from build123d import *

# Parameters (mm, degrees)
BOSS_EXTRUDE1_DEPTH = 22.86
SKETCH2_R           = 3.175
CUT_EXTRUDE1_DEPTH  = 50.737325059
SKETCH3_R           = 4.365625
CUT_EXTRUDE2_DEPTH  = 23.622


with BuildPart() as part:
    # Sketch1 → Boss-Extrude1 (new body)
    with BuildSketch(Plane(origin=(0, 0, 0), x_dir=(1, 0, 0), z_dir=(0, 1, 0))):
        Polygon((-11.176, -25.4), (-8.89, -25.4), (-8.89, 25.4), (8.89, 25.4), (8.89, -25.4), (11.176, -25.4), (11.176, 38.1), (-11.176, 38.1), align=None)
    extrude(amount=BOSS_EXTRUDE1_DEPTH)

    # Sketch2 → Cut-Extrude1 (cut, through all)
    with BuildSketch(Plane(origin=(11.176, 0, 0), x_dir=(0, 0, -1), z_dir=(1, 0, 0))):
        with Locations((-12.7, 11.43)):
            Circle(SKETCH2_R)
    extrude(amount=-CUT_EXTRUDE1_DEPTH, mode=Mode.SUBTRACT)

    # Sketch3 → Cut-Extrude2 (cut)
    with BuildSketch(Plane(origin=(0, 0, -38.1), x_dir=(-1, 0, 0), z_dir=(0, 0, -1))):
        with Locations((0, 11.43)):
            Circle(SKETCH3_R)
    extrude(amount=-CUT_EXTRUDE2_DEPTH, mode=Mode.SUBTRACT)


solid = part.part
CAD build for the part. Positions are in the model's coordinates, mm. A direction names the side the tool comes from. Give positions to 0.01 mm unless a question says otherwise; leave off trailing zeros. Order: outer loops, then holes, each group sorted by start corner. A loop starts at its lowest first (then second) coordinate and runs counter-clockwise, first axis right, second up. Notation, with made-up numbers: (15.5, 43) -> (40.5, 43) arc R31 ccw to (40.5, 74) -> close; hole circle Ø1 at (-17.75, 78.25). An arc over 180 degrees is marked (long way). Return JSON: item names as keys, results as strings.
Q1. Saw through at A-A (z = 12.7). Write the cut outline in (x, y) (3 decimals), then the cut area to 3 significant figures.
Working result:
{"outline": "(-11.176, 0) -> (-8.89, 0) -> (-8.89, 8.255) -> (-11.176, 8.255) -> close; (-11.176, 14.605) -> (-8.89, 14.605) -> (-8.89, 22.86) -> (-11.176, 22.86) -> close; (8.89, 0) -> (11.176, 0) -> (11.176, 8.255) -> (8.89, 8.255) -> close; (8.89, 14.605) -> (11.176, 14.605) -> (11.176, 22.86) -> (8.89, 22.86) -> close", "area": "75.5 mm²"}
Q2. Saw through at C-C (x = 0). Write the cut outline in (y, z).
Working result:
{"outline": "(0, -38.1) -> (7.06, -38.1) -> (7.06, -25.4) -> (0, -25.4) -> close; (15.8, -38.1) -> (22.86, -38.1) -> (22.86, -25.4) -> (15.8, -25.4) -> close"}
Q3. Saw through at D-D (z = 4.5). Write the cut outline in (x, y), then the cut area to 3 significant figures.
Working result:
{"outline": "(-11.18, 0) -> (-8.89, 0) -> (-8.89, 22.86) -> (-11.18, 22.86) -> close; (8.89, 0) -> (11.18, 0) -> (11.18, 22.86) -> (8.89, 22.86) -> close", "area": "105 mm²"}
Q4. Mould opens along Y. For faces 1 (the face through (0, 22.86, -28)), 2 (the face through (-10.02, 12.38, 9.67)), 3 (the face through (8.89, 11, 0)) say: pulls with the +Y half, pulls with the -Y half, needs draft (parallel to the pull), parting line crosses it, or undercut.
Working result:
{"face 1": "pulls with the +Y half", "face 2": "undercut", "face 3": "needs draft"}
Q5. Drill centre lines: line 1 (Y direction, x = -10.15, z = 12.7) (3 decimals); line 2 (Y direction, x = 0, z = -32.25); line 3 (X direction, y = 1.75, z = 0). Where is each one in solid material? Low to high.
Working result:
{"line 1": "0 to 8.255, 14.605 to 22.86", "line 2": "0 to 7.06, 15.8 to 22.86", "line 3": "-11.18 to -8.89, 8.89 to 11.18"}
Q6. Which spindle directions (+Z, -Z, +X, -X, +Y, -Y) get a long thin tool onto all of the face, cutting with end or side? Do faces 4 (the face through (-10, 11, 25.4)), 5 (the face through (4, 9, -25.4)). Say none if no direction does.
Working result:
{"face 4": "+Z, +X, -X, +Y, -Y", "face 5": "+Z, +Y, -Y"}
Q7. Saw through at B-B (y = 11.43). Write the cut outline in (x, z) (3 decimals), then the cut area to 3 significant figures.
Working result:
{"outline": "(-11.176, -38.1) -> (-4.366, -38.1) -> (-4.366, -25.4) -> (-8.89, -25.4) -> (-8.89, 9.525) -> (-11.176, 9.525) -> close; (-11.176, 15.875) -> (-8.89, 15.875) -> (-8.89, 25.4) -> (-11.176, 25.4) -> close; (4.366, -38.1) -> (11.176, -38.1) -> (11.176, 9.525) -> (8.89, 9.525) -> (8.89, -25.4) -> (4.366, -25.4) -> close; (8.89, 15.875) -> (11.176, 15.875) -> (11.176, 25.4) -> (8.89, 25.4) -> close", "area": "376 mm²"}
Q8. Flat gauge pin, fed straight in: pin 1 (8 mm diameter, centred on x = -1, y = 17.5, fed in from +Z). Where does the tip first touch, or does it go through?
Working result:
{"pin 1": "z = -25.4"}
